The model under review builds one solid part; all positions refer to its coordinate system, in mm. A direction names the side the tool comes from. Round coordinates to 2 decimals unless told otherwise and drop trailing zeros. Write each loop counter-clockwise with the first axis right and the second up, starting at its lowest first coordinate (ties: lowest second). Pieces come first, ordered by that corner, then holes. Notation, with made-up numbers: M 34.5,22 L 72.5,22 A10 cw 72.5,37 Z; hole C 68.5,57.5 d3. An arc over 180 degrees is marked long. Write item = value, one per line. Start each with the question number.
Item 1: Take a section at B-B, the plane y = 4. Give the boundary of the cut face in (x, z), plus the area to 3 significant figures.
Item 2: The part is to be moulded in two halves that separate along X. For faces 3 (the flat face through (-100, 76, 2)), 4 (the flat face through (-53.3, 95.7, 1.5)), say which applies: +X half, -X half, draft (parallel to the pull), parting line (faces both ways), or undercut.
Item 3: Take a section at D-D, the plane z = -3.5. Give the boundary of the cut face in (x, y).
Item 4: Take a section at A-A, the plane y = 77. Give the boundary of the cut face in (x, z), plus the area to 4 significant figures.
Item 5: To check wall thickness, follow line 1 along Y through (x, z) = (-96, 2.55); line 2 along Y through (x, z) = (-52, 2.2); line 3 along Y through (x, z) = (-50, 0.5). State the ranges of each line that lie inside material, in increasing order.
Item 6: For pin 1 Ø3.5 at (x, y) = (-4, 137) entering from -Z; pin 2 Ø8 at (x, y) = (-96, 137) entering from +Z; pin 3 Ø6.5 at (x, y) = (-51.5, 151.5) entering from -Z; pin 4 Ø3 at (x, z) = (-20, -3) entering from +Y, all flat-tipped, find the tip position at first contact; note any pin that passes through.
Item 7: Tool access review of faces 1 (the flat face through (-51.3, 2.7, 1.5)), 2 (the cylindrical face through (-4.761, 135.536, 2.732)): name each direction out of +Z, -Z, +X, -X, +Y, -Y from which nothing blocks a thin tool from reaching the whole face with its end or side.
Item 8: Take a section at C-C, the plane x = -85. Give the boundary of the cut face in (y, z).
from build123d import *

# Parameters (mm, degrees)
SKETCH1_W                     = 154
SKETCH1_H                     = 100
BOSS_EXTRUDE1_DEPTH           = 4
SKETCH2_R                     = 1.65
CUT_EXTRUDE1_DEPTH            = 184.66273438
SKETCH3_R                     = 7.5
BOSS_EXTRUDE2_DEPTH           = 6
BOSS_EXTRUDE2_DRAFT           = 15
BOSS_EXTRUDE2_PROFILE_2_DEPTH = 6
BOSS_EXTRUDE2_PROFILE_2_DRAFT = 15
BOSS_EXTRUDE2_PROFILE_3_DEPTH = 6
BOSS_EXTRUDE2_PROFILE_3_DRAFT = 15
BOSS_EXTRUDE2_PROFILE_4_DEPTH = 6
BOSS_EXTRUDE2_PROFILE_4_DRAFT = 15
SKETCH4_R                     = 3
CUT_EXTRUDE2_DEPTH            = 1.5


with BuildPart() as part:
    # Sketch1 → Boss-Extrude1 (new body)
    with BuildSketch(Plane(origin=(0, 0, 0), x_dir=(0, 1, 0), z_dir=(0, 0, 1))):
        with Locations((77, 50)):
            Rectangle(SKETCH1_W, SKETCH1_H)
    extrude(amount=BOSS_EXTRUDE1_DEPTH)

    # Sketch2 → Cut-Extrude1 (cut, through all)
    with BuildSketch(Plane(origin=(0, 0, 0), x_dir=(1, 0, 0), z_dir=(0, 0, -1))):
        with Locations(Location((-4, -77, 0), (0, 0, 180))):
            Circle(SKETCH2_R)
        with Locations(Location((-4, -17, 0), (0, 0, 180))):
            Circle(SKETCH2_R)
        with Locations(Location((-4, -137, 0), (0, 0, 180))):
            Circle(SKETCH2_R)
        with Locations(Location((-96, -137, 0), (0, 0, 180))):
            Circle(SKETCH2_R)
        with Locations(Location((-96, -77, 0), (0, 0, 180))):
            Circle(SKETCH2_R)
        with Locations(Location((-96, -17, 0), (0, 0, 180))):
            Circle(SKETCH2_R)
        with Locations(Location((-52, -97, 0), (0, 0, 180))):
            Circle(SKETCH2_R)
        with Locations(Location((-52, -57, 0), (0, 0, 180))):
            Circle(SKETCH2_R)
        with Locations(Location((-50, -4, 0), (0, 0, 180))):
            Circle(SKETCH2_R)
        with Locations(Location((-50, -150, 0), (0, 0, 180))):
            Circle(SKETCH2_R)
    extrude(amount=-CUT_EXTRUDE1_DEPTH, mode=Mode.SUBTRACT)


with BuildPart() as boss_extrude2_tool:
    # Sketch3 → Boss-Extrude2 (with draft: the straight prism first)
    with BuildSketch(Plane(origin=(0, 0, 0), x_dir=(1, 0, 0), z_dir=(0, 0, -1))):
        with Locations((-85, -15)):
            Circle(SKETCH3_R)
    extrude(amount=BOSS_EXTRUDE2_DEPTH)
    # Boss-Extrude2: the draft: its side faces are tilted about the plane it starts from
    boss_extrude2_sides = [boss_extrude2_tool.faces().sort_by_distance(p)[0] for p in [
        (-92.5, 15, -3),
    ]]
    draft(boss_extrude2_sides, Plane(origin=(0, 0, 0), x_dir=(1, 0, 0), z_dir=(0, 0, -1)), BOSS_EXTRUDE2_DRAFT)


with BuildPart() as part_1:
    add(part.part)

    # Boss-Extrude2: add boss_extrude2_tool
    add(boss_extrude2_tool.part)


with BuildPart() as boss_extrude2_profile_2_tool:
    # Sketch3 → Boss-Extrude2 profile 2 (with draft: the straight prism first)
    with BuildSketch(Plane(origin=(0, 0, 0), x_dir=(1, 0, 0), z_dir=(0, 0, -1))):
        with Locations((-15, -15)):
            Circle(SKETCH3_R)
    extrude(amount=BOSS_EXTRUDE2_PROFILE_2_DEPTH)
    # Boss-Extrude2 profile 2: the draft: its side faces are tilted about the plane it starts from
    boss_extrude2_profile_2_sides = [boss_extrude2_profile_2_tool.faces().sort_by_distance(p)[0] for p in [
        (-22.5, 15, -3),
    ]]
    draft(boss_extrude2_profile_2_sides, Plane(origin=(0, 0, 0), x_dir=(1, 0, 0), z_dir=(0, 0, -1)), BOSS_EXTRUDE2_PROFILE_2_DRAFT)


with BuildPart() as part_2:
    add(part_1.part)

    # Boss-Extrude2 profile 2: add boss_extrude2_profile_2_tool
    add(boss_extrude2_profile_2_tool.part)


with BuildPart() as boss_extrude2_profile_3_tool:
    # Sketch3 → Boss-Extrude2 profile 3 (with draft: the straight prism first)
    with BuildSketch(Plane(origin=(0, 0, 0), x_dir=(1, 0, 0), z_dir=(0, 0, -1))):
        with Locations((-15, -139)):
            Circle(SKETCH3_R)
    extrude(amount=BOSS_EXTRUDE2_PROFILE_3_DEPTH)
    # Boss-Extrude2 profile 3: the draft: its side faces are tilted about the plane it starts from
    boss_extrude2_profile_3_sides = [boss_extrude2_profile_3_tool.faces().sort_by_distance(p)[0] for p in [
        (-22.5, 139, -3),
    ]]
    draft(boss_extrude2_profile_3_sides, Plane(origin=(0, 0, 0), x_dir=(1, 0, 0), z_dir=(0, 0, -1)), BOSS_EXTRUDE2_PROFILE_3_DRAFT)


with BuildPart() as part_3:
    add(part_2.part)

    # Boss-Extrude2 profile 3: add boss_extrude2_profile_3_tool
    add(boss_extrude2_profile_3_tool.part)


with BuildPart() as boss_extrude2_profile_4_tool:
    # Sketch3 → Boss-Extrude2 profile 4 (with draft: the straight prism first)
    with BuildSketch(Plane(origin=(0, 0, 0), x_dir=(1, 0, 0), z_dir=(0, 0, -1))):
        with Locations((-85, -139)):
            Circle(SKETCH3_R)
    extrude(amount=BOSS_EXTRUDE2_PROFILE_4_DEPTH)
    # Boss-Extrude2 profile 4: the draft: its side faces are tilted about the plane it starts from
    boss_extrude2_profile_4_sides = [boss_extrude2_profile_4_tool.faces().sort_by_distance(p)[0] for p in [
        (-92.5, 139, -3),
    ]]
    draft(boss_extrude2_profile_4_sides, Plane(origin=(0, 0, 0), x_dir=(1, 0, 0), z_dir=(0, 0, -1)), BOSS_EXTRUDE2_PROFILE_4_DRAFT)


with BuildPart() as part_4:
    add(part_3.part)

    # Boss-Extrude2 profile 4: add boss_extrude2_profile_4_tool
    add(boss_extrude2_profile_4_tool.part)

    # Sketch4 → Cut-Extrude2 (cut)
    with BuildSketch(Plane(origin=(0, 0, 0), x_dir=(1, 0, 0), z_dir=(0, 0, -1))):
        with Locations(Location((-96, -17, 0), (0, 0, 180))):
            Circle(SKETCH4_R)
        with Locations(Location((-4, -17, 0), (0, 0, 180))):
            Circle(SKETCH4_R)
        with Locations(Location((-4, -77, 0), (0, 0, 180))):
            Circle(SKETCH4_R)
        with Locations(Location((-96, -77, 0), (0, 0, 180))):
            Circle(SKETCH4_R)
        with Locations(Location((-96, -137, 0), (0, 0, 180))):
            Circle(SKETCH4_R)
        with Locations(Location((-4, -137, 0), (0, 0, 180))):
            Circle(SKETCH4_R)
        with Locations(Location((-52, -57, 0), (0, 0, 180))):
            Circle(SKETCH4_R)
        with Locations(Location((-52, -97, 0), (0, 0, 180))):
            Circle(SKETCH4_R)
        with Locations(Location((-50, -4, 0), (0, 0, 180))):
            Circle(SKETCH4_R)
        with Locations(Location((-50, -150, 0), (0, 0, 180))):
            Circle(SKETCH4_R)
    extrude(amount=-CUT_EXTRUDE2_DEPTH, mode=Mode.SUBTRACT)


solid = part_4.part
Response values:
q1.outline = M -100,0 L -53,0 L -53,1.5 L -51.65,1.5 L -51.65,4 L -100,4 Z; M -48.35,1.5 L -47,1.5 L -47,0 L 0,0 L 0,4 L -48.35,4 Z
q1.area = 383 mm2
q2.face_3 = -X half
q2.face_4 = undercut
q3.outline = C -85,15 d13.12; C -85,139 d13.12; C -15,15 d13.12; C -15,139 d13.12
q4.outline = M -100,0 L -99,0 L -99,1.5 L -97.65,1.5 L -97.65,4 L -100,4 Z; M -94.35,1.5 L -93,1.5 L -93,0 L -7,0 L -7,1.5 L -5.65,1.5 L -5.65,4 L -94.35,4 Z; M -2.35,1.5 L -1,1.5 L -1,0 L 0,0 L 0,4 L -2.35,4 Z
q4.area = 365.5 mm2
q5.line_1 = 0 to 15.35, 18.65 to 75.35, 78.65 to 135.35, 138.65 to 154
q5.line_2 = 0 to 55.35, 58.65 to 95.35, 98.65 to 154
q5.line_3 = 0 to 1, 7 to 54.76, 59.24 to 94.76, 99.24 to 147, 153 to 154
q6.pin_1 = 1.5
q6.pin_2 = 4
q6.pin_3 = 0
q6.pin_4 = 144.82
q7.face_1 = -Z
q7.face_2 = +Z, -Z
q8.outline = M 0,0 L 7.5,0 L 9.11,-6 L 20.89,-6 L 22.5,0 L 131.5,0 L 133.11,-6 L 144.89,-6 L 146.5,0 L 154,0 L 154,4 L 0,4 Z
